```python
from build123d import *

# Parameters (mm, degrees)
SKETCH1_W           = 177.8
SKETCH1_H           = 76.2
BOSS_EXTRUDE1_DEPTH = 19.05
CUT_EXTRUDE1_DEPTH  = 3
SKETCH3_W           = 14.5
SKETCH3_H           = 14.5
SKETCH3_W_2         = 75.5
SKETCH3_H_2         = 6.35
CUT_EXTRUDE2_DEPTH  = 99.042962522
SKETCH4_R           = 3.5
CUT_EXTRUDE3_DEPTH  = 99.578509321
FILLET1_R           = 3.175
SKETCH5_R           = 6.25
CUT_EXTRUDE4_DEPTH  = 12.7
SKETCH6_W           = 3.175
SKETCH6_H           = 3.18
SKETCH6_W_2         = 3.18
CUT_EXTRUDE5_DEPTH  = 3
FILLET2_R           = 1.5875
FILLET3_R           = 1.59
FILLET4_R           = 1.5875
FILLET5_R           = 1.59
CUT_EXTRUDE6_DEPTH  = 35
CUT_EXTRUDE7_DEPTH  = 35


with BuildPart() as part:
    # Sketch1 → Boss-Extrude1 (new body)
    with BuildSketch(Plane(origin=(0, 0, 0), x_dir=(1, 0, 0), z_dir=(0, 1, 0))):
        Rectangle(SKETCH1_W, SKETCH1_H)
    extrude(amount=-BOSS_EXTRUDE1_DEPTH)

    # Sketch2 → Cut-Extrude1 (cut)
    with BuildSketch(Plane(origin=(0, 0, 0), x_dir=(1, 0, 0), z_dir=(0, 1, 0))):
        Polygon((37.75, 9.75), (82.75, 9.75), (82.75, -9.75), (37.75, -9.75), (37.75, -29.25), (-37.75, -29.25), (-37.75, -9.75), (-82.75, -9.75), (-82.75, 9.75), (-37.75, 9.75), (-37.75, 29.25), (37.75, 29.25), align=None)
    extrude(amount=-CUT_EXTRUDE1_DEPTH, mode=Mode.SUBTRACT)

    # Sketch3 → Cut-Extrude2 (cut, through all)
    with BuildSketch(Plane(origin=(0, -3, 0), x_dir=(1, 0, 0), z_dir=(0, 1, 0))):
        Rectangle(SKETCH3_W, SKETCH3_H)
        with Locations((0, 26.075)):
            Rectangle(SKETCH3_W_2, SKETCH3_H_2)
        with Locations((0, -26.075)):
            Rectangle(SKETCH3_W_2, SKETCH3_H_2)
    extrude(amount=-CUT_EXTRUDE2_DEPTH, mode=Mode.SUBTRACT)

    # Sketch4 → Cut-Extrude3 (cut, through all)
    with BuildSketch(Plane(origin=(0, 0, 0), x_dir=(1, 0, 0), z_dir=(0, 1, 0))):
        with Locations(Location((-76.2, 25.4, 0), (0, 0, 270))):
            Circle(SKETCH4_R)
        with Locations(Location((76.2, 25.4, 0), (0, 0, 270))):
            Circle(SKETCH4_R)
        with Locations(Location((76.2, -25.4, 0), (0, 0, 270))):
            Circle(SKETCH4_R)
        with Locations(Location((-76.2, -25.4, 0), (0, 0, 270))):
            Circle(SKETCH4_R)
    extrude(amount=-CUT_EXTRUDE3_DEPTH, mode=Mode.SUBTRACT)

    # Fillet1
    fillet1_edges = [part.edges().sort_by_distance(p)[0] for p in [
        (82.75, -1.5, -9.75),
        (82.75, -1.5, 9.75),
        (-82.75, -1.5, 9.75),
        (-82.75, -1.5, -9.75),
    ]]
    fillet(fillet1_edges, radius=FILLET1_R)

    # Sketch5 → Cut-Extrude4 (cut)
    with BuildSketch(Plane(origin=(0, 0, 0), x_dir=(1, 0, 0), z_dir=(0, 1, 0))):
        with Locations(Location((-76.2, -25.4, 0), (0, 0, 270))):
            Circle(SKETCH5_R)
        with Locations(Location((-76.2, 25.4, 0), (0, 0, 270))):
            Circle(SKETCH5_R)
        with Locations(Location((76.2, 25.4, 0), (0, 0, 270))):
            Circle(SKETCH5_R)
        with Locations(Location((76.2, -25.4, 0), (0, 0, 270))):
            Circle(SKETCH5_R)
    extrude(amount=-CUT_EXTRUDE4_DEPTH, mode=Mode.SUBTRACT)

    # Sketch6 → Cut-Extrude5 (cut)
    with BuildSketch(Plane(origin=(0, 0, 0), x_dir=(1, 0, 0), z_dir=(0, 1, 0))):
        with Locations((-36.1625, 30.84)):
            Rectangle(SKETCH6_W, SKETCH6_H)
        with Locations((36.16, 30.84)):
            Rectangle(SKETCH6_W_2, SKETCH6_H)
        with Locations((36.16, -30.84)):
            Rectangle(SKETCH6_W_2, SKETCH6_H)
        with Locations((-36.1625, -30.84)):
            Rectangle(SKETCH6_W, SKETCH6_H)
    extrude(amount=-CUT_EXTRUDE5_DEPTH, mode=Mode.SUBTRACT)

    # Fillet2
    fillet2_edges = [part.edges().sort_by_distance(p)[0] for p in [
        (-37.75, -1.5, -32.43),
        (-34.575, -1.5, -32.43),
    ]]
    fillet(fillet2_edges, radius=FILLET2_R - 0.0001)  # a hair under: the kernel refuses the full size

    # Fillet3
    fillet3_edges = [part.edges().sort_by_distance(p)[0] for p in [
        (37.75, -1.5, -32.43),
        (34.57, -1.5, -32.43),
    ]]
    fillet(fillet3_edges, radius=FILLET3_R - 0.0001)  # a hair under: the kernel refuses the full size

    # Fillet4
    fillet4_edges = [part.edges().sort_by_distance(p)[0] for p in [
        (-37.75, -1.5, 32.43),
        (-34.575, -1.5, 32.43),
    ]]
    fillet(fillet4_edges, radius=FILLET4_R - 0.0001)  # a hair under: the kernel refuses the full size

    # Fillet5
    fillet5_edges = [part.edges().sort_by_distance(p)[0] for p in [
        (37.75, -1.5, 32.43),
        (34.57, -1.5, 32.43),
    ]]
    fillet(fillet5_edges, radius=FILLET5_R - 0.0001)  # a hair under: the kernel refuses the full size

    # Sketch8 → Cut-Extrude6 (cut)
    with BuildSketch(Plane(origin=(0, -3, 0), x_dir=(1, 0, 0), z_dir=(0, 1, 0))):
        with BuildLine():
            Line((-75.75, 5.5), (-75.75, -5.5))
            ThreePointArc((-75.75, -5.5), (-78.75, -8.5), (-81.75, -5.5))
            Line((-81.75, -5.5), (-81.75, 5.5))
            ThreePointArc((-81.75, 5.5), (-78.75, 8.5), (-75.75, 5.5))
        make_face()
    extrude(amount=-CUT_EXTRUDE6_DEPTH, mode=Mode.SUBTRACT)

    # Sketch9 → Cut-Extrude7 (cut)
    with BuildSketch(Plane(origin=(0, -3, 0), x_dir=(1, 0, 0), z_dir=(0, 1, 0))):
        with BuildLine():
            Line((81.75, 5.5), (81.75, -5.5))
            ThreePointArc((81.75, -5.5), (78.75, -8.5), (75.75, -5.5))
            Line((75.75, -5.5), (75.75, 5.5))
            ThreePointArc((75.75, 5.5), (78.75, 8.5), (81.75, 5.5))
        make_face()
    extrude(amount=-CUT_EXTRUDE7_DEPTH, mode=Mode.SUBTRACT)


solid = part.part
```
The listing builds one solid part. Answer for the finished solid, in the listing's coordinates (mm). A direction names the side the tool comes from. Round coordinates to 2 decimals unless told otherwise and drop trailing zeros. Write each loop counter-clockwise with the first axis right and the second up, starting at its lowest first coordinate (ties: lowest second). Pieces come first, ordered by that corner, then holes. Notation, with made-up numbers: (-29, 56) -> (-15, 56) arc R25 cw to (-15, 79) -> close; hole circle Ø9 at (-20, 63). An arc over 180 degrees is marked (long way). Answer as a JSON object with one key per item and string values. Group by question number.
Q1. Section B-B (y = -15.5) is taken. Count the separate pieces of the cut face and the enclosed holes in it, plus the area to 3 significant figures.
Q2. Determine the mould class of faces 3 (the face through (-88.9, -9, 1)), 4 (the face through (-1, -19.05, -9)), 5 (the face through (81.8, -1.52, -8.84)) for opening direction X: pulls with the +X half, pulls with the -X half, needs draft (parallel to the pull), parting line crosses it, or undercut.
Q3. Section C-C (x = -67) is taken. Write down the section's boundary in (y, z).
Q4. Section D-D (z = -15) is taken. Write down the section's boundary in (x, y), plus the area to 3 significant figures.
Q5. Section A-A (z = -25.4) is taken. Write down the section's boundary in (x, y), plus the area to 3 significant figures.
Q6. Each of these flat-tipped pins is pushed along its axis until it touches: pin 1 Ø8 at (x, z) = (-76.2, 25.4) entering from +Y; pin 2 Ø20 at (x, z) = (-76.2, 25.4) entering from -Y; pin 3 Ø1.5 at (x, z) = (-29, -25) entering from -Y; pin 4 Ø5 at (x, z) = (18, -7) entering from +Y. Where does it stop, or does it pass through?
Q7. Which of the six approach directions +Z, -Z, +X, -X, +Y, -Y give full straight-line access (tool end or side, diameter ignored) to faces 1 (the face through (-59, -1, -9.75)), 2 (the face through (-1, -11, 22.9))?
Q8. Straight lines are drawn through the part: line 1 along Z through (x, y) = (-24, -16.25); line 2 along X through (y, z) = (-10, -25.4); line 3 along Z through (x, y) = (7, -8.5). For each, find the intervals that lie inside material, in ascending order.
Check values:
{
 "1": {"separate pieces": "1", "enclosed holes": "9", "area": "12,000 mm^2"},
 "2": {"face 3": "pulls with the -X half", "face 4": "needs draft", "face 5": "undercut"},
 "3": {"outline": "(-19.05, -38.1) -> (0, -38.1) -> (0, -9.75) -> (-3, -9.75) -> (-3, 9.75) -> (0, 9.75) -> (0, 38.1) -> (-19.05, 38.1) -> close"},
 "4": {"outline": "(-88.9, -19.05) -> (88.9, -19.05) -> (88.9, 0) -> (37.75, 0) -> (37.75, -3) -> (-37.75, -3) -> (-37.75, 0) -> (-88.9, 0) -> close", "area": "3,160 mm^2"},
 "5": {"outline": "(-88.9, -19.05) -> (-79.7, -19.05) -> (-79.7, -12.7) -> (-82.45, -12.7) -> (-82.45, 0) -> (-88.9, 0) -> close; (-72.7, -19.05) -> (-37.75, -19.05) -> (-37.75, 0) -> (-69.95, 0) -> (-69.95, -12.7) -> (-72.7, -12.7) -> close; (37.75, -19.05) -> (72.7, -19.05) -> (72.7, -12.7) -> (69.95, -12.7) -> (69.95, 0) -> (37.75, 0) -> close; (79.7, -19.05) -> (88.9, -19.05) -> (88.9, 0) -> (82.45, 0) -> (82.45, -12.7) -> (79.7, -12.7) -> close", "area": "1,540 mm^2"},
 "6": {"pin 1": "y = -12.7", "pin 2": "y = -19.05", "pin 3": "through", "pin 4": "y = -3"},
 "7": {"face 1": "+Y", "face 2": "+Y, -Y"},
 "8": {"line 1": "-38.1 to -29.25, -22.9 to 22.9, 29.25 to 38.1", "line 2": "-88.9 to -82.45, -69.95 to -37.75, 37.75 to 69.95, 82.45 to 88.9", "line 3": "-38.1 to -29.25, -22.9 to -7.25, 7.25 to 22.9, 29.25 to 38.1"}
}
